```python
from build123d import *
from build123d.topology import SkipClean

# Parameters (mm, degrees)
BOSS_EXTRUDE1_DEPTH     = 2
FINGERGRIP_DEPTH        = 0.3
BOSS_EXTRUDE2_DEPTH     = 2
REVOLVE1_ANGLE          = 180
CUT_EXTRUDE3_DEPTH      = 24.23093064
CUT_EXTRUDE3_DEPTH_BACK = 24.23093064
BOSS_EXTRUDE6_DEPTH     = 1.5
SKETCH24_R              = 1.9
SCREW_THREADS_DEPTH     = 3
SCREW_HEAD_REACH        = 24.63
SKETCH25_R              = 3.5
WALL1_DEPTH             = 1.5
WALL2_DEPTH             = 1.5


with BuildPart() as part:
    # Sketch1 → Boss-Extrude1 (new body)
    with BuildSketch(Plane.XY):
        with BuildLine():
            Line((-4, -10), (4, -10))
            ThreePointArc((4, -10), (5.414213562, -9.414213562), (6, -8))
            Line((6, -8), (6, 6))
            Line((6, 6), (3.305891799, 20.36857707))
            ThreePointArc((3.305891799, 20.36857707), (2.6174191, 21.539018216), (1.340147425, 22))
            Line((1.340147425, 22), (-1.340147425, 22))
            ThreePointArc((-1.340147425, 22), (-2.6174191, 21.539018216), (-3.305891799, 20.36857707))
            Line((-3.305891799, 20.36857707), (-6, 6))
            Line((-6, 6), (-6, -8))
            ThreePointArc((-6, -8), (-5.414213562, -9.414213562), (-4, -10))
        make_face()
    extrude(amount=BOSS_EXTRUDE1_DEPTH)

    # Sketch8 → FingerGrip (cut)
    with BuildSketch(Plane(origin=(0, 0, 0), x_dir=(-1, 0, 0), z_dir=(0, 0, -1))):
        with BuildLine():
            Line((-4, -4), (4, -4))
            ThreePointArc((4, -4), (4.75, -4.75), (4, -5.5))
            Line((4, -5.5), (-4, -5.5))
            ThreePointArc((-4, -5.5), (-4.75, -4.75), (-4, -4))
        make_face()
        with BuildLine():
            Line((-4, -7), (4, -7))
            ThreePointArc((4, -7), (4.75, -7.75), (4, -8.5))
            Line((4, -8.5), (-4, -8.5))
            ThreePointArc((-4, -8.5), (-4.75, -7.75), (-4, -7))
        make_face()
    extrude(amount=-FINGERGRIP_DEPTH, mode=Mode.SUBTRACT)

    # Sketch2 → Boss-Extrude2 (add)
    with BuildSketch(Plane(origin=(0, 0.340762895, 3.894937707), x_dir=(-1, 0, 0), z_dir=(0, 0.08715574274765835, 0.9961946980917455))):
        with BuildLine():
            Line((6, -5.802856703), (-6, -5.802856703))
            Line((-6, -5.802856703), (-3.305891799, -20.116756999))
            add(Edge.make_bspline(
                [(-3.305891799, -20.116756999), (-3, -21.741971873), (-1.340147425, -21.741971873)],
                knots=[3.326940604, 3.326940604, 3.326940604, 4.71238898, 4.71238898, 4.71238898], degree=2, weights=[1, 0.769509108, 1]))
            Line((-1.340147425, -21.741971873), (1.340147425, -21.741971873))
            add(Edge.make_bspline(
                [(1.340147425, -21.741971873), (3, -21.741971873), (3.305891799, -20.116756999)],
                knots=[4.71238898, 4.71238898, 4.71238898, 6.097837357, 6.097837357, 6.097837357], degree=2, weights=[1, 0.769509108, 1]))
            Line((3.305891799, -20.116756999), (6, -5.802856703))
        make_face()
    extrude(amount=-BOSS_EXTRUDE2_DEPTH)

    # Sketch9 → Revolve1 (revolve)
    with BuildSketch(Plane(origin=(0, 0.340762895, 3.894937707), x_dir=(1, 0, 0), z_dir=(0, 0.08715574274765836, 0.9961946980917457))):
        with BuildLine():
            Line((-2, 16.741971873), (2, 16.741971873))
            ThreePointArc((2, 16.741971873), (0, 14.741971873), (-2, 16.741971873))
        make_face()
    revolve(axis=Axis((0, 17.01902651, 2.435778714), (-1, 0, 0)), revolution_arc=REVOLVE1_ANGLE)

    # Sketch11 → Cut-Extrude3 (cut, two sides)
    with SkipClean():  # the faces are left unmerged after this step: merging them gives an invalid solid
        with BuildSketch(Plane(origin=(0, 0, 0), x_dir=(0, 0, -1), z_dir=(1, 0, 0))) as cut_extrude3_sk:
            Polygon((-4.435231088, 17.065826116), (-2.847274196, 18.976236633), (-5.75514434, 18.976236633), align=None)
        extrude(amount=CUT_EXTRUDE3_DEPTH, mode=Mode.SUBTRACT)
        extrude(cut_extrude3_sk.sketch, amount=-CUT_EXTRUDE3_DEPTH_BACK, mode=Mode.SUBTRACT)

    # Sketch17 → Boss-Extrude6 (add)
    with SkipClean():  # the faces are left unmerged after this step: merging them gives an invalid solid
        with BuildSketch(Plane(origin=(0, 0.764171798, 4.333833624), x_dir=(1, 0, 0), z_dir=(0, 0.1736481776669307, 0.984807753012208))):
            with BuildLine():
                Line((-4, 7.440012187), (-4, -2.559987813))
                ThreePointArc((-4, -2.559987813), (-3.414213562, -3.974201376), (-2, -4.559987813))
                Line((-2, -4.559987813), (2, -4.559987813))
                ThreePointArc((2, -4.559987813), (3.414213562, -3.974201376), (4, -2.559987813))
                Line((4, -2.559987813), (4, 7.440012187))
                Line((4, 7.440012187), (-4, 7.440012187))
            make_face()
        extrude(amount=-BOSS_EXTRUDE6_DEPTH)

    # Sketch23 for ChannelLoft → ChannelLoft section 0
    with SkipClean():  # the faces are left unmerged after this step: merging them gives an invalid solid
        with BuildSketch(Plane(origin=(0, 0.764171798, 4.333833624), x_dir=(1, 0, 0), z_dir=(0, 0.1736481776669307, 0.984807753012208))):
            with BuildLine():
                Line((-4, 5.440012187), (-4, -2.559987813))
                # circular arc as an exact rational Bezier (weights 1, cos(half-angle), 1)
                Bezier((-4, -2.559987813), (-4, -4.559987813), (-2, -4.559987813), weights=[1, 0.707106781, 1])
                Line((-2, -4.559987813), (2, -4.559987813))
                Bezier((2, -4.559987813), (4, -4.559987813), (4, -2.559987813), weights=[1, 0.707106781, 1])
                Line((4, -2.559987813), (4, 5.440012187))
                Line((4, 5.440012187), (-4, 5.440012187))
            make_face()
        # Sketch19 for ChannelLoft → ChannelLoft section 1
        with BuildSketch(Plane(origin=(0, 1.024644064, 5.811045254), x_dir=(1, 0, 0), z_dir=(0, 0.1736481776669307, 0.9848077530122081))):
            with BuildLine():
                Line((-3.25, 5.440012187), (-3.25, -2.559987813))
                Bezier((-3.25, -2.559987813), (-3.25, -4.559987813), (-1.25, -4.559987813), weights=[1, 0.707106781, 1])
                Line((-1.25, -4.559987813), (1.25, -4.559987813))
                Bezier((1.25, -4.559987813), (3.25, -4.559987813), (3.25, -2.559987813), weights=[1, 0.707106781, 1])
                Line((3.25, -2.559987813), (3.25, 5.440012187))
                Line((3.25, 5.440012187), (-3.25, 5.440012187))
            make_face()
        loft()

    # Sketch24 → Screw Threads (cut)
    with SkipClean():  # the faces are left unmerged after this step: merging them gives an invalid solid
        with BuildSketch(Plane(origin=(0, 1.024644064, 5.811045254), x_dir=(1, 0, 0), z_dir=(0, 0.17364817766693072, 0.9848077530122081))):
            with Locations(Location((0, 0.440012187, 0), (0, 0, 270))):
                Circle(SKETCH24_R)
        extrude(amount=-SCREW_THREADS_DEPTH, mode=Mode.SUBTRACT)

    # Screw Head: up to this plane
    with SkipClean():  # the faces are left unmerged after this step: merging them gives an invalid solid
        screw_head_end = Plane(origin=(1.340147425, 20, 0), z_dir=(0, 0, 1))
        # Sketch25 → Screw Head (cut, up to the surface)
        with BuildSketch(Plane(origin=(0, 0.503699531, 2.856621995), x_dir=(-1, 0, 0), z_dir=(0, -0.1736481776669307, -0.9848077530122081)), mode=Mode.PRIVATE) as screw_head_sk1:
            with Locations(Location((0, 0.440012187, 0), (0, 0, 90))):
                Circle(SKETCH25_R)
        screw_head_tool1 = split(extrude(screw_head_sk1.sketch, amount=SCREW_HEAD_REACH, mode=Mode.PRIVATE), bisect_by=screw_head_end, keep=Keep.BOTH, mode=Mode.PRIVATE)
        add(screw_head_tool1.solids().sort_by_distance((0, 0.937027, 2.780215))[0], mode=Mode.SUBTRACT)

    # Sketch26 → Wall1 (add)
    with SkipClean():  # the faces are left unmerged after this step: merging them gives an invalid solid
        with BuildSketch(Plane(origin=(6, 0, 0), x_dir=(0, 0, -1), z_dir=(1, 0, 0))):
            Polygon((-2, 6), (-3.389185421, 6.121537976), (-2, -8), align=None)
        extrude(amount=-WALL1_DEPTH)

    # Sketch27 → Wall2 (add)
    with SkipClean():  # the faces are left unmerged after this step: merging them gives an invalid solid
        with BuildSketch(Plane.ZY.offset(6)):
            Polygon((3.389185421, 6.121537976), (2, 6), (2, -8), align=None)
        extrude(amount=-WALL2_DEPTH)


solid = part.part
```
Input: part model. Units: mm. Frame: model coordinates. A direction names the side the tool comes from. Give positions to 0.01 mm unless a question says otherwise; leave off trailing zeros. Order: outer loops, then holes, each group sorted by start corner. A loop starts at its lowest first (then second) coordinate and runs counter-clockwise, first axis right, second up.
1. Pin query (flat end, axial travel): pin 1 (1 mm diameter, centred on x = 4, z = 4.5, fed in from -Y); pin 2 (2 mm diameter, centred on x = -2.5, y = 17, fed in from +Z); pin 3 (0.8 mm diameter, centred on y = 0.5, z = 3.5, fed in from +X). Return the tip coordinate at first contact, or that it passes through.
Derived:
pin 1: stops at y = -3.16
pin 2: stops at z = 3.76
pin 3: stops at x = 4
2. Mould query, pull axis Z, two halves, no side actions, for faces 1 (the flat face through (0, 22, 1)), 2 (the flat face through (0, -4, 2)), 3 (the flat face through (2.1, 2.8, 5.5)). Classes: released by +Z, released by -Z, zero draft, split by the parting line, or undercut.
Derived:
face 1: zero draft
face 2: undercut
face 3: released by +Z
3. Section C-C on y = -4.75. Return the cut outline in (x, z), and give its area (3 significant figures).
Derived:
outline: (-6, 0) - (-4.75, 0) - (-4.75, 0.3) - (4.75, 0.3) - (4.75, 0) - (6, 0) - (6, 2.32) - (4.5, 2.32) - (4.5, 2) - (-4.5, 2) - (-4.5, 2.32) - (-6, 2.32) - close
area: 22.1 mm2
4. Reachability of faces 4 (the flat face through (-4.634, 13.285, 0.986)), 5 (the flat face through (-4, 2, 3)), 6 (the flat face through (-5.26, -1.038, 2.685)) from +Z, -Z, +X, -X, +Y, -Y: full face, straight path, thin tool, end or side. Return the list, or none.
Derived:
face 4: -Z, -X, +Y
face 5: +Z, -Y
face 6: +Z, -X, -Y
5. Material intervals for L1, parallel to Y at x = -1.25, z = 3.75; L2, parallel to Z at x = 2.5, y = 19; L3, parallel to Y at x = -3, z = 0.75, sorted ascending.
Derived:
L1: y = -3.97 to -0.34, 2.56 to 6.19, 16.18 to 17.86
L2: z = 0 to 2.26
L3: y = -10 to -1.25, 2.41 to 21.12
6. Section A-A on y = 18. Return the cut outline in (x, z).
Derived:
outline: (-3.76, 2.35) - (-3.75, 2) - (-3.75, 0) - (3.75, 0) - (3.75, 2) - (3.76, 2.35) - (1.74, 2.35) arc R1.74 ccw to (1.24, 3.66) - (-1.24, 3.66) arc R1.74 ccw to (-1.74, 2.35) - close
7. Section B-B on y = 1.5. Give the number of separate pieces and of enclosed holes in the cut face, and give its area (3 significant figures).
Derived:
separate pieces: 4
enclosed holes: 0
area: 25.1 mm2
